Input: part model. Units: mm. Frame: model coordinates. A direction names the side the tool comes from. Give positions to 0.01 mm unless a question says otherwise; leave off trailing zeros. Write each loop counter-clockwise with the first axis right and the second up, starting at its lowest first coordinate (ties: lowest second). Pieces come first, ordered by that corner, then holes. Notation, with made-up numbers: (-32, -14) - (6, -14) arc R27 cw to (6, 18) - close; hole circle Ø11 at (55, 87.5). An arc over 180 degrees is marked (long way). Use a Markdown table: item, result. Add a question column.
1. Set-up query: faces 1 (the flat face through (13.7, -338, 5)), 2 (the flat face through (-18.3, -309, 15)), 3 (the flat face through (40, -275.947, 5)). Return all of +Z, -Z, +X, -X, +Y, -Y with unobstructed straight access to the full face (end or side cutting, diameter ignored); none if empty.
2. Pin query (flat end, axial travel): pin 1 (10 mm diameter, centred on x = 4, y = -279.5, fed in from +Z); pin 2 (11 mm diameter, centred on x = 34.5, z = 4.5, fed in from -Y); pin 3 (11 mm diameter, centred on x = 52, z = 6, fed in from +Y). Return the tip coordinate at first contact, or that it passes through.
3. Section query B-B, the plane z = 25.5. Return loops of the section in (x, y).
4. Section query C-C, the plane x = -30.5. Return loops of the section in (y, z).
5. Section query A-A, the plane x = 49.5. Return loops of the section in (y, z), plus the area to 3 significant figures.
6. Mould query, pull axis Z, two halves, no side actions, for faces 4 (the cylindrical face through (-11.377, -280.14, 21.064)), 5 (the flat face through (-17.8, -284, 42)), 6 (the cylindrical face through (6.71, -273.1, 4.93)), 7 (the flat face through (-19, -283, 50)). Classes: released by +Z, released by -Z, zero draft, split by the parting line, or undercut.
7. Section query D-D, the plane z = 6. Return loops of the section in (x, y).
8. Material intervals for probe 1 along Z at (x, y) = (-23.5, -283.5); probe 2 along X at (y, z) = (-295.5, 17.5); probe 3 along Z at (x, y) = (-41.5, -328), sorted ascending.
```python
from build123d import *

# Parameters (mm, degrees)
BOSS_EXTRUDE1_DEPTH = 10
SKETCH1_3_W         = 31
SKETCH1_3_H         = 55.042796233
BOSS_EXTRUDE2_DEPTH = 19
BOSS_EXTRUDE3_DEPTH = 3
SKETCH8_W           = 25
SKETCH8_H           = 18
BOSS_EXTRUDE4_DEPTH = 40
CUT_EXTRUDE2_DEPTH  = 101.93603831
SKETCH11_R          = 1.5
CUT_EXTRUDE3_DEPTH  = 365.137190302
SKETCH12_R          = 5
CUT_EXTRUDE4_DEPTH  = 21.5
SKETCH13_R          = 4.5
CUT_EXTRUDE5_DEPTH  = 359.488203344
SKETCH14_R          = 3
CUT_EXTRUDE6_DEPTH  = 359.488203344


with BuildPart() as part:
    # Sketch1 → Boss-Extrude1 (new body)
    with BuildSketch(Plane.XY):
        with BuildLine():
            ThreePointArc((3.70003333, -250.511159837), (0.771101142, -243.440092025), (-6.29996667, -240.511159837))
            Line((-6.29996667, -240.511159837), (-39.29996667, -240.511159837))
            ThreePointArc((-39.29996667, -240.511159837), (-46.371034482, -243.440092025), (-49.29996667, -250.511159837))
            Line((-49.29996667, -250.511159837), (-49.29996667, -340.06501156))
            ThreePointArc((-49.29996667, -340.06501156), (-46.371034482, -347.136079372), (-39.29996667, -350.06501156))
            Line((-39.29996667, -350.06501156), (3.70003333, -350.06501156))
            ThreePointArc((3.70003333, -350.06501156), (10.771101142, -347.136079372), (13.70003333, -340.06501156))
            Line((13.70003333, -340.06501156), (13.70003333, -335.947269399))
            Line((13.70003333, -335.947269399), (66.09296194, -335.947269399))
            Line((66.09296194, -335.947269399), (66.09296194, -275.947269399))
            Line((66.09296194, -275.947269399), (13.70003333, -275.947269399))
            ThreePointArc((13.70003333, -275.947269399), (6.628965518, -273.018337211), (3.70003333, -265.947269399))
            Line((3.70003333, -265.947269399), (3.70003333, -250.511159837))
        make_face()
    extrude(amount=BOSS_EXTRUDE1_DEPTH)

    # Sketch1<3> → Boss-Extrude2 (add)
    with BuildSketch(Plane.XY):
        with Locations((-33.79996667, -298.425871282)):
            Rectangle(SKETCH1_3_W, SKETCH1_3_H)
    extrude(amount=BOSS_EXTRUDE2_DEPTH)

    # Sketch2 → Boss-Extrude3 (add)
    with BuildSketch(Plane.XY.offset(19)):
        Polygon((-44.79996667, -321.447269399), (-44.79996667, -274.447269399), (-20.79996667, -274.447269399), (-20.79996667, -292.147269399), (-18.29996667, -292.147269399), (-18.29996667, -270.904473166), (-49.29996667, -270.904473166), (-49.29996667, -325.947269399), (-18.29996667, -325.947269399), (-18.29996667, -320.947269399), (-20.79996667, -320.947269399), (-20.79996667, -321.447269399), align=None)
    extrude(amount=BOSS_EXTRUDE3_DEPTH)

    # Sketch8 → Boss-Extrude4 (add)
    with BuildSketch(Plane.XY.offset(10)):
        with Locations((-8.29996667, -283.447269399)):
            Rectangle(SKETCH8_W, SKETCH8_H)
    extrude(amount=BOSS_EXTRUDE4_DEPTH)

    # Sketch9 → Cut-Extrude2 (cut, through all)
    with BuildSketch(Plane.XZ.offset(292.447269399)):
        Polygon((-17.79996667, 50), (4.20003333, 10), (4.20003333, 50), align=None)
    extrude(amount=-CUT_EXTRUDE2_DEPTH, mode=Mode.SUBTRACT)

    # Sketch11 → Cut-Extrude3 (cut, through all)
    with BuildSketch(Plane.ZY.offset(20.79996667)):
        with Locations(Location((43.5, -282.447269399, 0), (0, 0, 270))):
            Circle(SKETCH11_R)
        with Locations(Location((25.5, -282.447269399, 0), (0, 0, 270))):
            Circle(SKETCH11_R)
    extrude(amount=-CUT_EXTRUDE3_DEPTH, mode=Mode.SUBTRACT)

    # Sketch12 → Cut-Extrude4 (cut)
    with BuildSketch(Plane(origin=(3.70003333, 0, 0), x_dir=(0, 0, -1), z_dir=(1, 0, 0))):
        with Locations(Location((-43.5, -282.447269399, 0), (0, 0, 90))):
            Circle(SKETCH12_R)
        with Locations(Location((-25.5, -282.447269399, 0), (0, 0, 90))):
            Circle(SKETCH12_R)
    extrude(amount=-CUT_EXTRUDE4_DEPTH, mode=Mode.SUBTRACT)

    # Sketch13 → Cut-Extrude5 (cut, through all)
    with BuildSketch(Plane.XY.offset(10)):
        with Locations((-19.49996667, -261.947269399)):
            Circle(SKETCH13_R)
        with Locations((-19.49996667, -333.947269399)):
            Circle(SKETCH13_R)
    extrude(amount=-CUT_EXTRUDE5_DEPTH, mode=Mode.SUBTRACT)

    # Sketch14 → Cut-Extrude6 (cut, through all)
    with BuildSketch(Plane.XY.offset(10)):
        with Locations((60.09296194, -282.697269399)):
            Circle(SKETCH14_R)
        with Locations((48.092961938, -282.697269399)):
            Circle(SKETCH14_R)
        with Locations(Location((60.09296194, -329.197269399, 0), (0, 0, 180))):
            Circle(SKETCH14_R)
        with Locations(Location((48.092961938, -329.197269399, 0), (0, 0, 180))):
            Circle(SKETCH14_R)
    extrude(amount=-CUT_EXTRUDE6_DEPTH, mode=Mode.SUBTRACT)


solid = part.part
```
Result sheet:
| question | item | result |
|---|---|---|
| 1 | face 1 | +Z, -Z, +X, -Y |
| 1 | face 2 | +Z, +X, -Y |
| 1 | face 3 | +Z, -Z, +X, +Y |
| 2 | pin 1 | stops at z = 19.45 |
| 2 | pin 2 | stops at y = -335.95 |
| 2 | pin 3 | stops at y = -275.95 |
| 3 | outline | (-20.8, -292.45) - (-4.32, -292.45) - (-4.32, -287.45) - (-17.8, -287.45) - (-17.8, -283.95) - (-20.8, -283.95) - close; (-20.8, -280.95) - (-17.8, -280.95) - (-17.8, -277.45) - (-4.32, -277.45) - (-4.32, -274.45) - (-20.8, -274.45) - close |
| 4 | outline | (-350.07, 0) - (-240.51, 0) - (-240.51, 10) - (-270.9, 10) - (-270.9, 22) - (-274.45, 22) - (-274.45, 19) - (-321.45, 19) - (-321.45, 22) - (-325.95, 22) - (-325.95, 10) - (-350.07, 10) - close |
| 5 | outline | (-335.95, 0) - (-331.85, 0) - (-331.85, 10) - (-335.95, 10) - close; (-326.55, 0) - (-285.35, 0) - (-285.35, 10) - (-326.55, 10) - close; (-280.05, 0) - (-275.95, 0) - (-275.95, 10) - (-280.05, 10) - close |
| 5 | area | 494 mm² |
| 6 | face 4 | undercut |
| 6 | face 5 | undercut |
| 6 | face 6 | zero draft |
| 6 | face 7 | released by +Z |
| 7 | outline | (-49.3, -340.07) arc R10 ccw to (-39.3, -350.07) - (3.7, -350.07) arc R10 ccw to (13.7, -340.07) - (13.7, -335.95) - (66.09, -335.95) - (66.09, -275.95) - (13.7, -275.95) arc R10 cw to (3.7, -265.95) - (3.7, -250.51) arc R10 ccw to (-6.3, -240.51) - (-39.3, -240.51) arc R10 ccw to (-49.3, -250.51) - close; hole circle Ø9 at (-19.5, -333.95); hole circle Ø9 at (-19.5, -261.95); hole circle Ø6 at (48.09, -329.2); hole circle Ø6 at (48.09, -282.7); hole circle Ø6 at (60.09, -329.2); hole circle Ø6 at (60.09, -282.7) |
| 8 | probe 1 | z = 0 to 19 |
| 8 | probe 2 | x = -49.3 to -18.3 |
| 8 | probe 3 | z = 0 to 10 |
